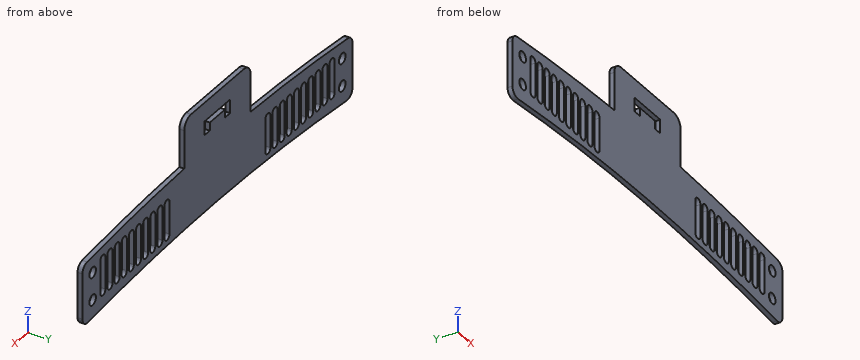
from build123d import *

# Parameters (mm, degrees)
SKETCH1_R           = 3.25
BOSS_EXTRUDE1_DEPTH = 3


with BuildPart() as part:
    # Sketch1 → Boss-Extrude1 (new body)
    with BuildSketch(Plane(origin=(0, 0, 0), x_dir=(1, 0, 0), z_dir=(0, 1, 0))):
        with BuildLine():
            Line((-10, 6.436614591), (-10, -21.493672684))
            ThreePointArc((-10, -21.493672684), (-8.711123408, -24.844428278), (-5.508974779, -26.467699692))
            ThreePointArc((-5.508974779, -26.467699692), (42.187344307, -30.432754781), (90, -32.579955692))
            Line((90, -32.579955692), (90, -56.029565828))
            ThreePointArc((90, -56.029565828), (91.918564772, -60.66139092), (96.550389863, -62.579955692))
            Line((96.550389863, -62.579955692), (148.449610137, -62.579955692))
            ThreePointArc((148.449610137, -62.579955692), (153.081435228, -60.66139092), (155, -56.029565828))
            Line((155, -56.029565828), (155, -32.579955692))
            ThreePointArc((155, -32.579955692), (202.812655693, -30.432754781), (250.508974779, -26.467699692))
            ThreePointArc((250.508974779, -26.467699692), (253.711123408, -24.844428278), (255, -21.493672684))
            Line((255, -21.493672684), (255, 6.436614591))
            ThreePointArc((255, 6.436614591), (253.346445742, 10.151624806), (249.479479641, 11.409446637))
            ThreePointArc((249.479479641, 11.409446637), (122.5, 4.781900515), (-4.479479641, 11.409446637))
            ThreePointArc((-4.479479641, 11.409446637), (-8.346445742, 10.151624806), (-10, 6.436614591))
        make_face()
        with Locations(Location((0, 0, 0), (0, 0, 270))):
            Circle(SKETCH1_R, mode=Mode.SUBTRACT)
        with Locations(Location((245, 0, 0), (0, 0, 270))):
            Circle(SKETCH1_R, mode=Mode.SUBTRACT)
        with Locations(Location((0, -17, 0), (0, 0, 270))):
            Circle(SKETCH1_R, mode=Mode.SUBTRACT)
        with Locations(Location((245, -17, 0), (0, 0, 270))):
            Circle(SKETCH1_R, mode=Mode.SUBTRACT)
        with BuildLine():
            Line((12.5, 0), (12.5, -20))
            ThreePointArc((12.5, -20), (10, -22.5), (7.5, -20))
            Line((7.5, -20), (7.5, 0))
            ThreePointArc((7.5, 0), (10, 2.5), (12.5, 0))
        make_face(mode=Mode.SUBTRACT)
        with BuildLine():
            Line((19.5, 0), (19.5, -20))
            ThreePointArc((19.5, -20), (17, -22.5), (14.5, -20))
            Line((14.5, -20), (14.5, 0))
            ThreePointArc((14.5, 0), (17, 2.5), (19.5, 0))
        make_face(mode=Mode.SUBTRACT)
        with BuildLine():
            Line((26.5, 0), (26.5, -20))
            ThreePointArc((26.5, -20), (24, -22.5), (21.5, -20))
            Line((21.5, -20), (21.5, 0))
            ThreePointArc((21.5, 0), (24, 2.5), (26.5, 0))
        make_face(mode=Mode.SUBTRACT)
        with BuildLine():
            Line((33.5, 0), (33.5, -20))
            ThreePointArc((33.5, -20), (31, -22.5), (28.5, -20))
            Line((28.5, -20), (28.5, 0))
            ThreePointArc((28.5, 0), (31, 2.5), (33.5, 0))
        make_face(mode=Mode.SUBTRACT)
        with BuildLine():
            Line((40.5, 0), (40.5, -20))
            ThreePointArc((40.5, -20), (38, -22.5), (35.5, -20))
            Line((35.5, -20), (35.5, 0))
            ThreePointArc((35.5, 0), (38, 2.5), (40.5, 0))
        make_face(mode=Mode.SUBTRACT)
        with BuildLine():
            Line((47.5, 0), (47.5, -20))
            ThreePointArc((47.5, -20), (45, -22.5), (42.5, -20))
            Line((42.5, -20), (42.5, 0))
            ThreePointArc((42.5, 0), (45, 2.5), (47.5, 0))
        make_face(mode=Mode.SUBTRACT)
        with BuildLine():
            Line((54.5, 0), (54.5, -20))
            ThreePointArc((54.5, -20), (52, -22.5), (49.5, -20))
            Line((49.5, -20), (49.5, 0))
            ThreePointArc((49.5, 0), (52, 2.5), (54.5, 0))
        make_face(mode=Mode.SUBTRACT)
        with BuildLine():
            Line((61.5, 0), (61.5, -20))
            ThreePointArc((61.5, -20), (59, -22.5), (56.5, -20))
            Line((56.5, -20), (56.5, 0))
            ThreePointArc((56.5, 0), (59, 2.5), (61.5, 0))
        make_face(mode=Mode.SUBTRACT)
        with BuildLine():
            Line((68.5, 0), (68.5, -20))
            ThreePointArc((68.5, -20), (66, -22.5), (63.5, -20))
            Line((63.5, -20), (63.5, 0))
            ThreePointArc((63.5, 0), (66, 2.5), (68.5, 0))
        make_face(mode=Mode.SUBTRACT)
        with BuildLine():
            Line((75.5, 0), (75.5, -20))
            ThreePointArc((75.5, -20), (73, -22.5), (70.5, -20))
            Line((70.5, -20), (70.5, 0))
            ThreePointArc((70.5, 0), (73, 2.5), (75.5, 0))
        make_face(mode=Mode.SUBTRACT)
        with BuildLine():
            Line((174.5, 0), (174.5, -20))
            ThreePointArc((174.5, -20), (172, -22.5), (169.5, -20))
            Line((169.5, -20), (169.5, 0))
            ThreePointArc((169.5, 0), (172, 2.5), (174.5, 0))
        make_face(mode=Mode.SUBTRACT)
        with BuildLine():
            Line((181.5, 0), (181.5, -20))
            ThreePointArc((181.5, -20), (179, -22.5), (176.5, -20))
            Line((176.5, -20), (176.5, 0))
            ThreePointArc((176.5, 0), (179, 2.5), (181.5, 0))
        make_face(mode=Mode.SUBTRACT)
        with BuildLine():
            Line((188.5, 0), (188.5, -20))
            ThreePointArc((188.5, -20), (186, -22.5), (183.5, -20))
            Line((183.5, -20), (183.5, 0))
            ThreePointArc((183.5, 0), (186, 2.5), (188.5, 0))
        make_face(mode=Mode.SUBTRACT)
        with BuildLine():
            Line((195.5, 0), (195.5, -20))
            ThreePointArc((195.5, -20), (193, -22.5), (190.5, -20))
            Line((190.5, -20), (190.5, 0))
            ThreePointArc((190.5, 0), (193, 2.5), (195.5, 0))
        make_face(mode=Mode.SUBTRACT)
        with BuildLine():
            Line((202.5, 0), (202.5, -20))
            ThreePointArc((202.5, -20), (200, -22.5), (197.5, -20))
            Line((197.5, -20), (197.5, 0))
            ThreePointArc((197.5, 0), (200, 2.5), (202.5, 0))
        make_face(mode=Mode.SUBTRACT)
        with BuildLine():
            Line((209.5, 0), (209.5, -20))
            ThreePointArc((209.5, -20), (207, -22.5), (204.5, -20))
            Line((204.5, -20), (204.5, 0))
            ThreePointArc((204.5, 0), (207, 2.5), (209.5, 0))
        make_face(mode=Mode.SUBTRACT)
        with BuildLine():
            Line((216.5, 0), (216.5, -20))
            ThreePointArc((216.5, -20), (214, -22.5), (211.5, -20))
            Line((211.5, -20), (211.5, 0))
            ThreePointArc((211.5, 0), (214, 2.5), (216.5, 0))
        make_face(mode=Mode.SUBTRACT)
        with BuildLine():
            Line((223.5, 0), (223.5, -20))
            ThreePointArc((223.5, -20), (221, -22.5), (218.5, -20))
            Line((218.5, -20), (218.5, 0))
            ThreePointArc((218.5, 0), (221, 2.5), (223.5, 0))
        make_face(mode=Mode.SUBTRACT)
        with BuildLine():
            Line((230.5, 0), (230.5, -20))
            ThreePointArc((230.5, -20), (228, -22.5), (225.5, -20))
            Line((225.5, -20), (225.5, 0))
            ThreePointArc((225.5, 0), (228, 2.5), (230.5, 0))
        make_face(mode=Mode.SUBTRACT)
        with BuildLine():
            Line((237.5, 0), (237.5, -20))
            ThreePointArc((237.5, -20), (235, -22.5), (232.5, -20))
            Line((232.5, -20), (232.5, 0))
            ThreePointArc((232.5, 0), (235, 2.5), (237.5, 0))
        make_face(mode=Mode.SUBTRACT)
        Polygon((115, -42.579955692), (115, -47.579955692), (130, -47.579955692), (130, -42.579955692), (135, -42.579955692), (135, -51.079955692), (110, -51.079955692), (110, -42.579955692), align=None, mode=Mode.SUBTRACT)
    extrude(amount=BOSS_EXTRUDE1_DEPTH)


solid = part.part
Can you work these out from the model? Positions are in its coordinate system, mm. Coordinates: 2 decimals unless noted, no trailing zeros. Write each loop counter-clockwise with the first axis right and the second up, starting at its lowest first coordinate (ties: lowest second). Pieces come first, ordered by that corner, then holes. Notation, with made-up numbers: (30.5, 62) - (34.5, 62) arc R14 cw to (34.5, 81) - close; hole circle Ø10 at (85, -30.5). An arc over 180 degrees is marked (long way). Return JSON: item names as keys, results as strings. Group by question number.
Item 1: I'm going to push a flat-ended pin straight in: pin 1 Ø5 at (x, z) = (143.5, 53) entering from -Y. Where does the tip first touch, or does it pass through?
Item 2: If we section it at B-B (x = 0): Write out the boundary of the cut face in (y, z).
Item 3: If we section it at A-A (x = 214): Write out the boundary of the cut face in (y, z).
Item 4: If we section it at C-C (z = 8): Count the separate pieces of the cut face and the enclosed holes in it, then the cut area to 3 significant figures.
Item 5: Please list where these lines run through material, in increasing order: probe 1 along X at (y, z) = (0.5, 43); probe 2 along Z at (x, y) = (124, 0.65); probe 3 along Z at (x, y) = (245, 1.4).
Return value:
{
 "1": {"pin 1": "stops at y = 0"},
 "2": {"outline": "(0, -10.95) - (3, -10.95) - (3, -3.25) - (0, -3.25) - close; (0, 3.25) - (3, 3.25) - (3, 13.75) - (0, 13.75) - close; (0, 20.25) - (3, 20.25) - (3, 27.02) - (0, 27.02) - close"},
 "3": {"outline": "(0, -8.22) - (3, -8.22) - (3, -2.5) - (0, -2.5) - close; (0, 22.5) - (3, 22.5) - (3, 29.67) - (0, 29.67) - close"},
 "4": {"separate pieces": "21", "enclosed holes": "0", "area": "495 mm^2"},
 "5": {"probe 1": "x = 90 to 110, 115 to 130, 135 to 155", "probe 2": "z = -4.78 to 47.58, 51.08 to 62.58", "probe 3": "z = -10.95 to -3.25, 3.25 to 13.75, 20.25 to 27.02"}
}
